from build123d import *

# Parameters (mm, degrees)
F0_W     = 122.5
F0_H     = 92.5
F0_R     = 13.25
F1_DEPTH = 1
F2_DEPTH = 2
F3_R     = 2.55
F4_DEPTH = 2.001


# Not quite as in the source:
# - a feature names something its author has since deleted; it is built from what else it names


with BuildPart() as f1:
    # F0 (on Top) → F1 (new body)
    with BuildSketch(Plane.XY):
        Rectangle(F0_W, F0_H)
        with Locations((-45, -30)):
            Circle(F0_R, mode=Mode.SUBTRACT)
        with Locations((-15, -30)):
            Circle(F0_R, mode=Mode.SUBTRACT)
        with Locations((15, -30)):
            Circle(F0_R, mode=Mode.SUBTRACT)
        with Locations((45, -30)):
            Circle(F0_R, mode=Mode.SUBTRACT)
        with Locations((-45, 0)):
            Circle(F0_R, mode=Mode.SUBTRACT)
        with Locations((-15, 0)):
            Circle(F0_R, mode=Mode.SUBTRACT)
        with Locations((-45, 30)):
            Circle(F0_R, mode=Mode.SUBTRACT)
        with Locations((-15, 30)):
            Circle(F0_R, mode=Mode.SUBTRACT)
        with Locations((15, 0)):
            Circle(F0_R, mode=Mode.SUBTRACT)
        with Locations((45, 0)):
            Circle(F0_R, mode=Mode.SUBTRACT)
        with Locations((15, 30)):
            Circle(F0_R, mode=Mode.SUBTRACT)
        with Locations((45, 30)):
            Circle(F0_R, mode=Mode.SUBTRACT)
        with Locations((-45, 30)):
            Circle(F0_R)
        with Locations((-15, 30)):
            Circle(F0_R)
        with Locations((15, 30)):
            Circle(F0_R)
        with Locations((45, 30)):
            Circle(F0_R)
        with Locations((45, 0)):
            Circle(F0_R)
        with Locations((-15, 0)):
            Circle(F0_R)
        with Locations((-45, 0)):
            Circle(F0_R)
        with Locations((15, 0)):
            Circle(F0_R)
        with Locations((15, -30)):
            Circle(F0_R)
        with Locations((-15, -30)):
            Circle(F0_R)
        with Locations((-45, -30)):
            Circle(F0_R)
        with Locations((45, -30)):
            Circle(F0_R)
    extrude(amount=F1_DEPTH)

    # F0 (on Top) → F2 (join)
    with BuildSketch(Plane.XY):
        Rectangle(F0_W, F0_H)
        with Locations((-45, -30)):
            Circle(F0_R, mode=Mode.SUBTRACT)
        with Locations((-15, -30)):
            Circle(F0_R, mode=Mode.SUBTRACT)
        with Locations((15, -30)):
            Circle(F0_R, mode=Mode.SUBTRACT)
        with Locations((45, -30)):
            Circle(F0_R, mode=Mode.SUBTRACT)
        with Locations((-45, 0)):
            Circle(F0_R, mode=Mode.SUBTRACT)
        with Locations((-15, 0)):
            Circle(F0_R, mode=Mode.SUBTRACT)
        with Locations((-45, 30)):
            Circle(F0_R, mode=Mode.SUBTRACT)
        with Locations((-15, 30)):
            Circle(F0_R, mode=Mode.SUBTRACT)
        with Locations((15, 0)):
            Circle(F0_R, mode=Mode.SUBTRACT)
        with Locations((45, 0)):
            Circle(F0_R, mode=Mode.SUBTRACT)
        with Locations((15, 30)):
            Circle(F0_R, mode=Mode.SUBTRACT)
        with Locations((45, 30)):
            Circle(F0_R, mode=Mode.SUBTRACT)
    extrude(amount=F2_DEPTH)

    # F3 (on face) → F4 (cut, through all)
    with BuildSketch(Plane.XY.offset(2)):
        with Locations((-57.2, 42.2)):
            Circle(F3_R)
        with Locations((57.2, 42.2)):
            Circle(F3_R)
        with Locations((-57.2, -42.2)):
            Circle(F3_R)
        with Locations((57.2, -42.2)):
            Circle(F3_R)
    extrude(amount=-F4_DEPTH, mode=Mode.SUBTRACT)


solid = f1.part
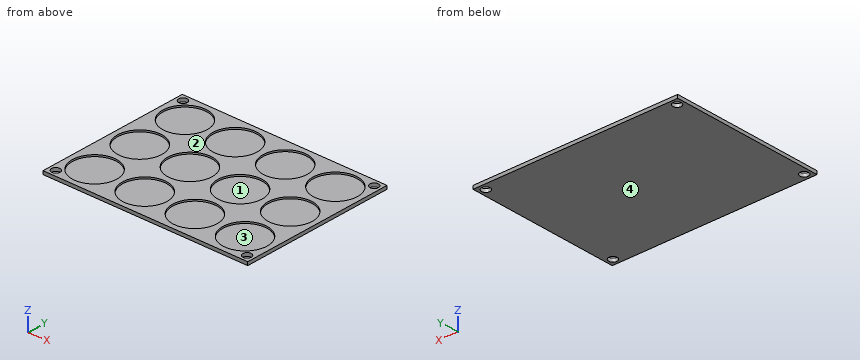
Design review of the part built by this model. Coordinates are the model's own, in mm. Face numbers are marked on the shaded views. A direction names the side the tool comes from. Coordinates: 2 decimals unless noted, no trailing zeros. Loops run counter-clockwise (first coordinate to the right, second up) from the corner with the lowest first, then second, coordinate; pieces in that order, holes last. Notation, with made-up numbers: (-11, -7) -> (14, -7) arc R19 ccw to (14, 23) -> close; hole circle Ø4 at (-31, 73.5). An arc over 180 degrees is marked (long way). Use a Markdown table: item, result. Add a question column.
Item 1: We need section A-A, the plane z = 1.4. Count the separate pieces of the cut face and the enclosed holes in it, and give its area (3 significant figures).
Item 2: Machinability: for the marked faces 1 and 2, which of the approach directions +Z, -Z, +X, -X, +Y, -Y give a long, thin tool a straight path to every point of the face, cutting with its end or side? Answer none if there is none.
Item 3: We need section B-B, the plane y = 37. Write out the cut boundary in (x, z).
Item 4: We need section C-C, the plane x = -15.5. Write out the cut boundary in (y, z), and give its area (3 significant figures).
Item 5: Clearance check with flat-ended pins moving along their axes: P1, Ø13, axis at x = -51.5, y = -31.5, coming from the +Z side; P2, Ø3, axis at x = -57.2, y = -42.2, coming from the +Z side. State where each tip first meets the part, or that it passes through.
Item 6: We need section D-D, the plane x = -52. Write out the cut boundary in (y, z), and give its area (4 significant figures).
Item 7: Wall thickness on L1, parallel to X at y = -30, z = 1.75; L2, parallel to Y at x = 15, z = 1.3; L3, parallel to Y at x = 57.2, z = 0.85: over which ranges is each line inside the solid? List them lowest first. Write a range as from..to.
Item 8: The part is to be moulded in two halves that separate along X. For the marked faces 3 and 4, say which applies: +X half, -X half, draft (parallel to the pull), parting line (faces both ways), or undercut.
Numbers:
| question | item | result |
|---|---|---|
| 1 | separate pieces | 1 |
| 1 | enclosed holes | 16 |
| 1 | area | 4,630 mm^2 |
| 2 | face 1 | +Z |
| 2 | face 2 | +Z, +X, -X, +Y, -Y |
| 3 | outline | (-61.25, 0) -> (61.25, 0) -> (61.25, 2) -> (56.25, 2) -> (56.25, 1) -> (33.75, 1) -> (33.75, 2) -> (26.25, 2) -> (26.25, 1) -> (3.75, 1) -> (3.75, 2) -> (-3.75, 2) -> (-3.75, 1) -> (-26.25, 1) -> (-26.25, 2) -> (-33.75, 2) -> (-33.75, 1) -> (-56.25, 1) -> (-56.25, 2) -> (-61.25, 2) -> close |
| 4 | outline | (-46.25, 0) -> (46.25, 0) -> (46.25, 2) -> (43.24, 2) -> (43.24, 1) -> (16.76, 1) -> (16.76, 2) -> (13.24, 2) -> (13.24, 1) -> (-13.24, 1) -> (-13.24, 2) -> (-16.76, 2) -> (-16.76, 1) -> (-43.24, 1) -> (-43.24, 2) -> (-46.25, 2) -> close |
| 4 | area | 106 mm^2 |
| 5 | P1 | stops at z = 1 |
| 5 | P2 | passes through |
| 6 | outline | (-46.25, 0) -> (46.25, 0) -> (46.25, 2) -> (41.25, 2) -> (41.25, 1) -> (18.75, 1) -> (18.75, 2) -> (11.25, 2) -> (11.25, 1) -> (-11.25, 1) -> (-11.25, 2) -> (-18.75, 2) -> (-18.75, 1) -> (-41.25, 1) -> (-41.25, 2) -> (-46.25, 2) -> close |
| 6 | area | 117.5 mm^2 |
| 7 | L1 | x = -61.25..-58.25, -31.75..-28.25, -1.75..1.75, 28.25..31.75, 58.25..61.25 |
| 7 | L2 | y = -46.25..-43.25, -16.75..-13.25, 13.25..16.75, 43.25..46.25 |
| 7 | L3 | y = -46.25..-44.75, -39.65..39.65, 44.75..46.25 |
| 8 | face 3 | undercut |
| 8 | face 4 | draft |
